CAD build for the part. Positions are in the model's coordinates, mm. Face numbers are marked on the shaded views. Give positions to 0.01 mm unless a question says otherwise; leave off trailing zeros. Write each loop counter-clockwise with the first axis right and the second up, starting at its lowest first coordinate (ties: lowest second). Pieces come first, ordered by that corner, then holes. Notation, with made-up numbers: (2, 6) - (13, 6) arc R36 cw to (13, 43) - close; hole circle Ø1 at (52, 0). An arc over 180 degrees is marked (long way). Write item = value, one per line. Start each with the question number.
```python
from build123d import *

# Parameters (mm, degrees)
F1_DEPTH = 31.75
F2_R     = 7.237328
F2_R_2   = 7.492319
F2_R_3   = 11.262041
F3_DEPTH = 76.2


with BuildPart() as f1:
    # F0 (on Front) → F1 (new body)
    with BuildSketch(Plane.XZ):
        Polygon((23.56123, 60.866501), (0, 36.814418), (0, 5.154018), (74.855983, 5.154018), (74.855983, 60.866501), align=None)
    extrude(amount=F1_DEPTH)

    # F2 (on face) → F3 (cut)
    with BuildSketch(Plane.XZ.offset(31.75)):
        with Locations((56.380846, 45.629557)):
            Circle(F2_R)
        with Locations((57.339922, 21.812528)):
            Circle(F2_R_2)
        with Locations((20.575382, 28.685898)):
            Circle(F2_R_3)
    extrude(amount=-F3_DEPTH, mode=Mode.SUBTRACT)


solid = f1.part
```
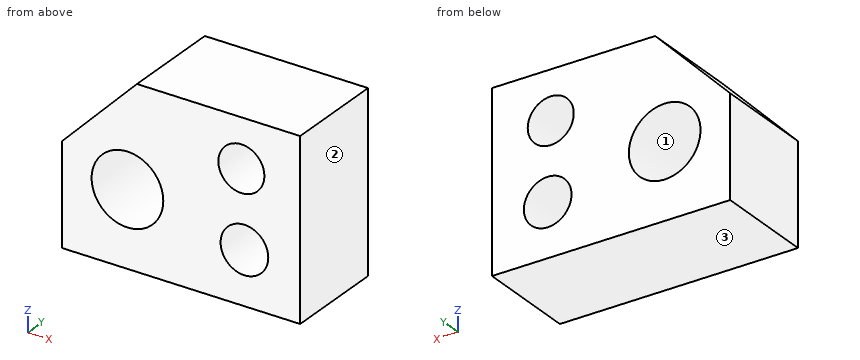
1. Cut at A-A (z = 41.5). Give the cut face in (x, y).
2. Mould opens along Z. For the marked faces 1, 2 and 3 say: +Z half, -Z half, draft (parallel to the pull), parting line (faces both ways), or undercut.
3. Cut at D-D (y = -8.5). Give the cut face in (x, z).
4. Cut at C-C (x = 16.5). Give the cut face in (y, z).
5. Cut at B-B (z = 26). Give the cut face in (x, y).
6. Wall check: line 1 along Z through (x, y) = (62.5, -4) (1 decimal); line 2 along X through (y, z) = (-7, 19.5); line 3 along Z through (x, y) = (62, -3.5). Give the ranges that are in metal, low to high.
Output:
q1.outline = (4.59, -31.75) - (50.44, -31.75) - (50.44, 0) - (4.59, 0) - close; (62.32, -31.75) - (74.86, -31.75) - (74.86, 0) - (62.32, 0) - close
q2.face_1 = undercut
q2.face_2 = draft
q2.face_3 = -Z half
q3.outline = (0, 5.15) - (74.86, 5.15) - (74.86, 60.87) - (23.56, 60.87) - (0, 36.81) - close; hole circle Ø22.52 at (20.58, 28.69); hole circle Ø14.47 at (56.38, 45.63); hole circle Ø14.98 at (57.34, 21.81)
q4.outline = (-31.75, 5.15) - (0, 5.15) - (0, 18.19) - (-31.75, 18.19) - close; (-31.75, 39.18) - (0, 39.18) - (0, 53.66) - (-31.75, 53.66) - close
q5.outline = (0, -31.75) - (9.64, -31.75) - (9.64, 0) - (0, 0) - close; (31.51, -31.75) - (51.13, -31.75) - (51.13, 0) - (31.51, 0) - close; (63.55, -31.75) - (74.86, -31.75) - (74.86, 0) - (63.55, 0) - close
q6.line_1 = 5.2 to 16.4, 27.2 to 41.8, 49.5 to 60.9
q6.line_2 = 0 to 14.06, 27.09 to 50.21, 64.47 to 74.86
q6.line_3 = 5.15 to 15.95, 27.68 to 41.07, 50.19 to 60.87
